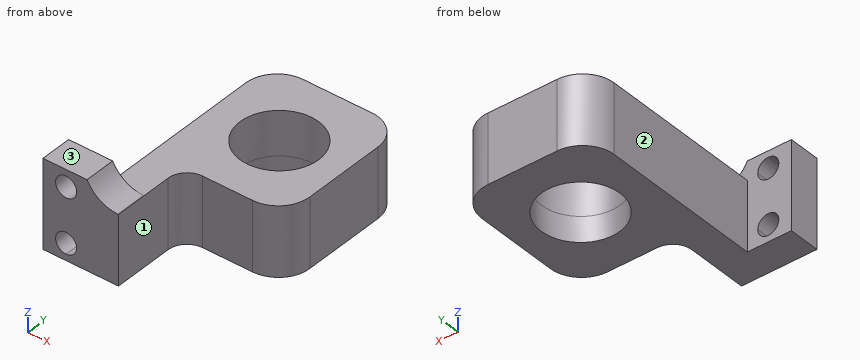
from build123d import *

# Parameters (mm, degrees)
F0_W         = 28
F0_H         = 36
F1_DEPTH     = 4
F2_R         = 6.25
F2_W         = 7
F2_H         = 31
F2_W_2       = 16
F2_H_2       = 12.7
F3_DEPTH     = 25
F4_W         = 7
F4_H         = 5
F4_R         = 6.25
F5_DEPTH     = 7
F6_DEPTH     = 10
F8_DEPTH     = 25
F9_R         = 5
F10_R        = 3
F11_T1_DEPTH = 5


# Not quite as in the source:
# - a fillet or chamfer that OpenCascade refuses, or shapes differently, is made with other operations: its cross-section is extruded or revolved along the edge and cut away or added


with BuildPart() as f1:
    # F0 (on Top) → F1 (new body)
    with BuildSketch(Plane.XY):
        with Locations((14, 18)):
            Rectangle(F0_W, F0_H)
    extrude(amount=F1_DEPTH)

    # F2 (on face) → F3 (cut)
    with BuildSketch(Plane.XY.offset(4)):
        with Locations((17.75, 24.35)):
            Circle(F2_R)
        with Locations((3.5, 20.5)):
            Rectangle(F2_W, F2_H)
        with Locations((20, 6.35)):
            Rectangle(F2_W_2, F2_H_2)
    extrude(amount=-F3_DEPTH, mode=Mode.SUBTRACT)

    # F4 (on face) → F5 (join)
    with BuildSketch(Plane.XY.offset(4)):
        with Locations((3.5, 2.5)):
            Rectangle(F4_W, F4_H)
        Polygon((7, 36), (7, 5), (7, 0), (12, 0), (12, 12.7), (28, 12.7), (28, 36), align=None)
        with Locations((17.75, 24.35)):
            Circle(F4_R, mode=Mode.SUBTRACT)
    extrude(amount=F5_DEPTH)

    # F4 (on face) → F6 (join)
    with BuildSketch(Plane.XY.offset(4)):
        with Locations((3.5, 2.5)):
            Rectangle(F4_W, F4_H)
    extrude(amount=F6_DEPTH)

    # F7 (on face) → F8 (cut)
    with BuildSketch(Plane.XZ):
        with BuildLine():
            ThreePointArc((3.675, 13), (2.4905961415, 10.1405961415), (5.35, 11.325))
            ThreePointArc((5.35, 11.325), (4.8594038585, 12.5094038585), (3.675, 13))
        make_face()
        with BuildLine():
            ThreePointArc((3.675, 1), (4.8594038585, 1.4905961415), (5.35, 2.675))
            ThreePointArc((5.35, 2.675), (2.4905961415, 3.8594038585), (3.675, 1))
        make_face()
    extrude(amount=-F8_DEPTH, mode=Mode.SUBTRACT)

    # F9
    f9_edges = [f1.edges().sort_by_distance(p)[0] for p in [
        (28, 36, 5.5),
        (7, 36, 5.5),
        (28, 12.7, 5.5),
    ]]
    fillet(f9_edges, radius=F9_R)

    # F10
    f10_edges = [f1.edges().sort_by_distance(p)[0] for p in [
        (12, 12.7, 5.5),
    ]]
    fillet(f10_edges, radius=F10_R)

    # F11: fillet of radius 5.5 on 1 edges, made by hand

    # F11_s2 → F11_t1 (join)
    with BuildSketch(Plane.XZ.offset(-5)):
        with BuildLine():
            ThreePointArc((11.8989794856, 11), (9.0266981623, 11.8095842402), (7, 14))
            Line((7, 14), (7, 11))
            Line((7, 11), (11.8989794856, 11))
        make_face()
    extrude(amount=F11_T1_DEPTH)


solid = f1.part
Model file for the job. Use its own axes, mm. Face numbers are marked on the shaded views. A direction names the side the tool comes from. Coordinates: 2 decimals unless noted, no trailing zeros. Order: outer loops, then holes, each group sorted by start corner. A loop starts at its lowest first (then second) coordinate and runs counter-clockwise, first axis right, second up. Notation, with made-up numbers: M -37,50.25 L -18,50.25 A15 ccw -18,58.25 Z; hole C 66,64.5 d1. An arc over 180 degrees is marked long. Return JSON: item names as keys, results as strings.
1. Tool access for the marked faces 1, 2 and 3: list every direction of +Z, -Z, +X, -X, +Y, -Y with a clear straight run to the whole face (end or side of a thin tool).
Ans:
{"face 1": "+Z, -Z, +X, -Y", "face 2": "+Z, -Z, -X, +Y", "face 3": "+Z, +X, -X, +Y, -Y"}
2. Saw through at D-D (z = 10.25). Give the cut face in (x, y).
Ans:
{"outline": "M 0,0 L 2.39,0 L 2.39,5 L 0,5 Z; M 4.96,0 L 12,0 L 12,9.7 A3 cw 15,12.7 L 23,12.7 A5 ccw 28,17.7 L 28,31 A5 ccw 23,36 L 12,36 A5 ccw 7,31 L 7,5 L 4.96,5 Z; hole C 17.75,24.35 d12.5"}
3. Drill centre lines: probe 1 along Y at (x, z) = (17.75, 9.75); probe 2 along Y at (x, z) = (19.5, 3.5); probe 3 along Z at (x, y) = (22.25, 33.5). Where is each one in solid material? Low to high.
Ans:
{"probe 1": "12.7 to 18.1, 30.6 to 36", "probe 2": "12.7 to 18.35, 30.35 to 36", "probe 3": "0 to 11"}
4. Saw through at B-B (x = 17.75). Give the cut face in (y, z), and give its area (3 significant figures).
Ans:
{"outline": "M 12.7,0 L 18.1,0 L 18.1,11 L 12.7,11 Z; M 30.6,0 L 36,0 L 36,11 L 30.6,11 Z", "area": "119 mm^2"}
5. Saw through at C-C (y = 24.35). Give the cut face in (x, z).
Ans:
{"outline": "M 7,0 L 11.5,0 L 11.5,11 L 7,11 Z; M 24,0 L 28,0 L 28,11 L 24,11 Z"}
6. Saw through at A-A (z = 5.25). Give the cut face in (x, y), and give its area (3 significant figures).
Ans:
{"outline": "M 0,0 L 12,0 L 12,9.7 A3 cw 15,12.7 L 23,12.7 A5 ccw 28,17.7 L 28,31 A5 ccw 23,36 L 12,36 A5 ccw 7,31 L 7,5 L 0,5 Z; hole C 17.75,24.35 d12.5", "area": "451 mm^2"}
7. Flat gauge pins, fed straight in: pin 1 (2 mm diameter, centred on x = 13.5, z = 2, fed in from -Y); pin 2 (12 mm diameter, centred on x = 15, y = 30.5, fed in from +Z); pin 3 (2 mm diameter, centred on x = 3.675, z = 11.325, fed in from +Y); pin 4 (2.5 mm diameter, centred on x = 17.5, z = 6, fed in from -Y). Where does each tip first touch, or does it go through?
Ans:
{"pin 1": "y = 11.36", "pin 2": "z = 11", "pin 3": "through", "pin 4": "y = 12.7"}
